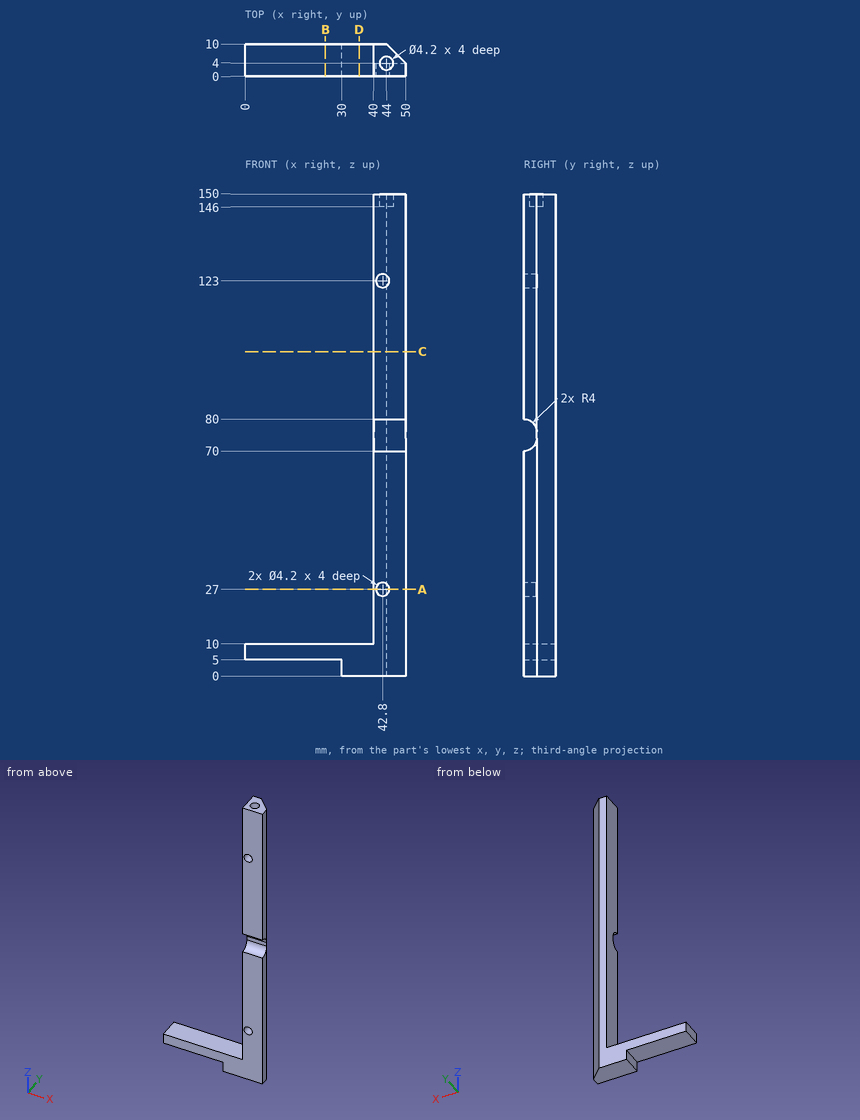
Source: three-view drawing plus pictorial views. Frame: mm from the lowest corner of the part. Give positions to 0.01 mm unless a question says otherwise; leave off trailing zeros. Order: outer loops, then holes, each group sorted by start corner. A loop starts at its lowest first (then second) coordinate and runs counter-clockwise, first axis right, second up. Notation, with made-up numbers: M 6,-6.5 L 40,-6.5 A17 ccw 40,2.5 Z; hole C -31.5,38.25 d5. An arc over 180 degrees is marked long. Return JSON: item names as keys, results as strings.
1) Section query C-C on z = 101. Output: boundary loops of the cut face in (x, y).
Taken from the geometry:
{"outline": "M 40,0 L 50,0 L 50,4 L 44,10 L 40,10 Z"}
2) Section query D-D on x = 35.5. Output: boundary loops of the cut face in (y, z).
Taken from the geometry:
{"outline": "M 0,0 L 10,0 L 10,10 L 0,10 Z"}
3) Section query A-A on z = 27. Output: boundary loops of the cut face in (x, y).
Taken from the geometry:
{"outline": "M 40,0 L 40.7,0 L 40.7,4 L 44.9,4 L 44.9,0 L 50,0 L 50,4 L 44,10 L 40,10 Z"}
4) Contact query for flat-ended pins moving along their axis: pin 1 (5 mm diameter, centred on x = 12.5, y = 3, fed in from +Z); pin 2 (4 mm diameter, centred on y = 5.5, z = 57.5, fed in from -X); pin 3 (0.6 mm diameter, centred on x = 43.5, z = 75, fed in from -Y). Output: stop coordinate, or through.
Taken from the geometry:
{"pin 1": "stops at z = 10", "pin 2": "stops at x = 40", "pin 3": "stops at y = 4"}
5) Line query: L1, parallel to X at y = 1, z = 144; L2, parallel to Y at x = 44, z = 148.1; L3, parallel to X at y = 1.2, z = 123. Output: solid intervals per line, ascending. Write a range as [from, to].
Taken from the geometry:
{"L1": "x = [40, 50]", "L2": "y = [0, 1.9], [6.1, 10]", "L3": "x = [40, 40.7], [44.9, 50]"}
6) Section query B-B on x = 25. Output: boundary loops of the cut face in (y, z).
Taken from the geometry:
{"outline": "M 0,5 L 10,5 L 10,10 L 0,10 Z"}
